Geometry check sheet. Reference: the model listing, model coordinates, mm. Round coordinates to 2 decimals unless told otherwise and drop trailing zeros. Write each loop counter-clockwise with the first axis right and the second up, starting at its lowest first coordinate (ties: lowest second). Pieces come first, ordered by that corner, then holes. Notation, with made-up numbers: M -25,23 L 32,23 A10 ccw 32,36 Z; hole C 41.25,4 d1. An arc over 180 degrees is marked long. One line per item, written item: value. Start each with the question number.
1. Section check A-A (x = 8). Record the boundary of the cut face in (y, z), and give its area (3 significant figures).
2. Section check B-B (z = 1.45). Record the boundary of the cut face in (x, y), and give its area (3 significant figures).
3. Release check for a two-part mould opening along Y. For faces 1 (the cylindrical face through (6.5, 0.07, 1.97)), 2 (the flat face through (-6, 2, 4)), 3 (the cylindrical face through (13.17, -2.19, 1.97)), 4 (the cylindrical face through (0.9, 12.1, 2)) record: pulls with the +Y half, pulls with the -Y half, needs draft (parallel to the pull), parting line crosses it, or undercut.
4. Depth check by flat-ended pin: P1, Ø1.8, axis at x = -8, y = 0, coming from the +Z side (1 decimal); P2, Ø1, axis at x = 7, z = 1, coming from the +Y side. Enter the tip coordinate at first touch or a pass-through.
5. Scan lines: probe 1 along Y at (x, z) = (0, 3.25); probe 2 along Y at (x, z) = (-8.5, 3.85); probe 3 along Y at (x, z) = (-8, 3.05). Record each from-to range of solid material in increasing order. Write a range as [from, to].
6. Section check C-C (y = 0). Record the boundary of the cut face in (x, z).
7. Section check D-D (y = 7). Record the boundary of the cut face in (x, z).
from build123d import *

# Parameters (mm, degrees)
SKETCH_1_R      = 1.5
SKETCH_1_R_2    = 2
SKETCH_1_R_3    = 3
EXTRUDE_1_DEPTH = 4


with BuildPart() as part:
    # 草图1 → 凸台-拉伸1 (new body)
    with BuildSketch(Plane.XY):
        with BuildLine():
            Line((-0.873328743, 11.958800349), (-21.485562705, 3.713906764))
            ThreePointArc((-21.485562705, 3.713906764), (-23.927825547, -0.756430085), (-20, -4))
            Line((-20, -4), (10.414213562, -4))
            ThreePointArc((10.414213562, -4), (13.18585216, -2.148050297), (12.535533906, 1.121320344))
            Line((12.535533906, 1.121320344), (2.36216363, 11.29469062))
            ThreePointArc((2.36216363, 11.29469062), (0.844040903, 12.112103444), (-0.873328743, 11.958800349))
        make_face()
        with Locations((0, 8)):
            Circle(SKETCH_1_R, mode=Mode.SUBTRACT)
        with Locations((8, 0)):
            Circle(SKETCH_1_R, mode=Mode.SUBTRACT)
        with Locations((-20, 0)):
            Circle(SKETCH_1_R_2, mode=Mode.SUBTRACT)
        Circle(SKETCH_1_R_3, mode=Mode.SUBTRACT)
        with Locations((-8, 0)):
            Circle(SKETCH_1_R, mode=Mode.SUBTRACT)
    extrude(amount=EXTRUDE_1_DEPTH)


solid = part.part
Result sheet:
1. outline: M -4,0 L -1.5,0 L -1.5,4 L -4,4 Z; M 1.5,0 L 5.66,0 L 5.66,4 L 1.5,4 Z
1. area: 26.6 mm2
2. outline: M -21.49,3.71 A4 ccw -20,-4 L 10.41,-4 A3 ccw 12.54,1.12 L 2.36,11.29 A3 ccw -0.87,11.96 Z; hole C -20,0 d4; hole C -8,0 d3; hole C 0,0 d6; hole C 0,8 d3; hole C 8,0 d3
2. area: 353 mm2
3. face 1: undercut
3. face 2: needs draft
3. face 3: parting line crosses it
3. face 4: pulls with the +Y half
4. P1: passes through
4. P2: stops at y = 7.16
5. probe 1: y = [-4, -3], [3, 6.5], [9.5, 12.16]
5. probe 2: y = [-4, -1.41], [1.41, 8.91]
5. probe 3: y = [-4, -1.5], [1.5, 9.11]
6. outline: M -24,0 L -22,0 L -22,4 L -24,4 Z; M -18,0 L -9.5,0 L -9.5,4 L -18,4 Z; M -6.5,0 L -3,0 L -3,4 L -6.5,4 Z; M 3,0 L 6.5,0 L 6.5,4 L 3,4 Z; M 9.5,0 L 13.24,0 L 13.24,4 L 9.5,4 Z
7. outline: M -13.27,0 L -1.12,0 L -1.12,4 L -13.27,4 Z; M 1.12,0 L 6.66,0 L 6.66,4 L 1.12,4 Z
